```python
from build123d import *

# Parameters (mm, degrees)
POCKET_DEPTH = 8.891


with BuildPart() as part:
    # Sketch → Revolution (revolve)
    with BuildSketch(Plane.XY):
        Polygon((0, 0), (0, 10.16), (1.905, 10.16), (1.905, 22.5425), (-1.27, 22.5425), (-1.27, 30.1625), (8.89, 30.1625), (8.89, 22.5425), (5.715, 22.5425), (5.715, 10.16), (7.62, 10.16), (7.62, 0), align=None)
    revolve(axis=Axis((0, 0, 0), (1, 0, 0)))

    # Sketch001 (on Face1 of Revolution) → Pocket (cut, through all)
    with BuildSketch(Plane(origin=(0, 0, 0), x_dir=(0, -1, 0), z_dir=(-1, 0, 0))):
        Polygon((0, 7.332348), (-6.35, 3.666174), (-6.35, -3.666174), (0, -7.332348), (6.35, -3.666174), (6.35, 3.666174), align=None)
    extrude(amount=-POCKET_DEPTH, mode=Mode.SUBTRACT)


solid = part.part
```
Source: CAD feature listing. Evaluate the final solid. Frame: model axes, mm. A direction names the side the tool comes from. Round coordinates to 2 decimals unless told otherwise and drop trailing zeros. Loops run counter-clockwise (first coordinate to the right, second up) from the corner with the lowest first, then second, coordinate; pieces in that order, holes last.
1. Ray query, L1, parallel to Z at x = 7.7, y = 0; L2, parallel to Z at x = 1.75, y = -4; L3, parallel to X at y = 11, z = -12 (3 decimals). Return the intervals inside material, ascending.
2. Section query A-A on x = 1. Give the number of separate pieces and of enclosed holes in the cut face, and give its area (3 significant figures).
3. Contact query for flat-ended pins moving along their axis: pin 1 (2 mm diameter, centred on x = 6.5, y = -18.5, fed in from -Z); pin 2 (6 mm diameter, centred on y = -5.5, z = -9, fed in from +X); pin 3 (3 mm diameter, centred on x = 5, y = -2, fed in from +Z); pin 4 (6 mm diameter, centred on x = 4.5, z = 1, fed in from -Y). Output: stop coordinate, or through.
4. Section query C-C on y = 4. Output: boundary loops of the cut face in (x, z) (3 decimals), and give its area (3 significant figures).
5. Mould query, pull axis Z, two halves, no side actions, for faces 4 (the cylindrical face through (7.28, -4.887, -22.006)), 5 (the flat face through (-1.27, -11, -20)), 6 (the cylindrical face through (3.881, -30.133, 1.326)). Classes: released by +Z, released by -Z, zero draft, split by the parting line, or undercut.
6. Access query for faces 1 (the flat face through (5.715, 5, -10)), 2 (the flat face through (3.757, 3.219, -5.474)), 3 (the flat face through (0, -7, 0)). Directions: +Z, -Z, +X, -X, +Y, -Y. A direction counts if a zero-diameter tool reaches every point of the face in a straight line with its end or side. Return the directions, or none.
7. Section query D-D on z = 8.5. Output: boundary loops of the cut face in (x, y) (3 decimals).
Answers below:
1. L1: z = -30.16 to -22.54, 22.54 to 30.16
1. L2: z = -29.9 to -22.18, -9.34 to -5.02, 5.02 to 9.34, 22.18 to 29.9
1. L3: x = 1.905 to 5.715
2. separate pieces: 2
2. enclosed holes: 2
2. area: 1,450 mm2
3. pin 1: stops at z = -24.57
3. pin 2: stops at x = 7.62
3. pin 3: stops at z = 30.16
3. pin 4: stops at y = -30.16
4. outline: (-1.27, -29.896) - (8.89, -29.896) - (8.89, -22.185) - (5.715, -22.185) - (5.715, -9.339) - (7.62, -9.339) - (7.62, -5.023) - (0, -5.023) - (0, -9.339) - (1.905, -9.339) - (1.905, -22.185) - (-1.27, -22.185) - close; (-1.27, 22.185) - (1.905, 22.185) - (1.905, 9.339) - (0, 9.339) - (0, 5.023) - (7.62, 5.023) - (7.62, 9.339) - (5.715, 9.339) - (5.715, 22.185) - (8.89, 22.185) - (8.89, 29.896) - (-1.27, 29.896) - close
4. area: 320 mm2
5. face 4: undercut
5. face 5: zero draft
5. face 6: split by the parting line
6. face 1: +X
6. face 2: +X, -X
6. face 3: -X
7. outline: (-1.27, -28.94) - (8.89, -28.94) - (8.89, -20.879) - (5.715, -20.879) - (5.715, -5.566) - (7.62, -5.566) - (7.62, 5.566) - (5.715, 5.566) - (5.715, 20.879) - (8.89, 20.879) - (8.89, 28.94) - (-1.27, 28.94) - (-1.27, 20.879) - (1.905, 20.879) - (1.905, 5.566) - (0, 5.566) - (0, -5.566) - (1.905, -5.566) - (1.905, -20.879) - (-1.27, -20.879) - close
